from build123d import *

# Parameters (mm, degrees)
SALIENTE_EXTRUIR2_DEPTH = 3.2


with BuildPart() as part:
    # Croquis1 → Saliente-Extruir2 (new body)
    with BuildSketch(Plane(origin=(0, 0, 0), x_dir=(1, 0, 0), z_dir=(0, 1, 0))):
        with BuildLine():
            Line((-16.5, 3), (16.5, 3))
            ThreePointArc((16.5, 3), (20.541451884, 3.596020491), (24.238791177, 5.333333333))
            ThreePointArc((24.238791177, 5.333333333), (30.841182772, 8.435677694), (38.058061137, 9.5))
            Line((38.058061137, 9.5), (57.5, 9.5))
            Line((57.5, 9.5), (57.5, -9.5))
            Line((57.5, -9.5), (38.058061137, -9.5))
            ThreePointArc((38.058061137, -9.5), (30.841182772, -8.435677694), (24.238791177, -5.333333333))
            ThreePointArc((24.238791177, -5.333333333), (20.541451884, -3.596020491), (16.5, -3))
            Line((16.5, -3), (-16.5, -3))
            ThreePointArc((-16.5, -3), (-20.541451884, -3.596020491), (-24.238791177, -5.333333333))
            ThreePointArc((-24.238791177, -5.333333333), (-30.841182772, -8.435677694), (-38.058061137, -9.5))
            Line((-38.058061137, -9.5), (-57.5, -9.5))
            Line((-57.5, -9.5), (-57.5, 9.5))
            Line((-57.5, 9.5), (-38.058061137, 9.5))
            ThreePointArc((-38.058061137, 9.5), (-30.841182772, 8.435677694), (-24.238791177, 5.333333333))
            ThreePointArc((-24.238791177, 5.333333333), (-20.541451884, 3.596020491), (-16.5, 3))
        make_face()
    extrude(amount=SALIENTE_EXTRUIR2_DEPTH)


solid = part.part
Verification items for the finished model (mm, model axes). A direction names the side the tool comes from. Give positions to 0.01 mm unless a question says otherwise; leave off trailing zeros. Order: outer loops, then holes, each group sorted by start corner. A loop starts at its lowest first (then second) coordinate and runs counter-clockwise, first axis right, second up. Notation, with made-up numbers: M -7.75,46 L -0.75,46 A20 cw -0.75,68 Z; hole C -28,-15.75 d11. An arc over 180 degrees is marked long. Answer as a JSON object with one key per item and string values. Group by question number.
1) Depth check by flat-ended pin: pin 1 Ø3 at (x, z) = (15.5, -6) entering from -Y. Enter the tip coordinate at first touch or a pass-through.
2) Cross-section at D-D (x = 19.5). Enter the section's corners in (y, z).
3) Cross-section at B-B (y = 1.25). Enter the section's corners in (x, z), then the cut area to 3 significant figures.
4) Cross-section at C-C (z = 7.75). Enter the section's corners in (x, y).
5) Cross-section at A-A (z = -6.75). Enter the section's corners in (x, y).
6) Scan lines: line 1 along X through (y, z) = (0.95, 5.5); line 2 along Z through (x, y) = (3, 2.65); line 3 along X through (y, z) = (2.8, 5). Record each from-to range of solid material in increasing order. Write a range as [from, to].
7) Access from +Z, -Z, +X, -X, +Y, -Y to the whole of each face (thin tool, end or side, straight path). Record for faces 1 (the face through (-30.743, 1.578, 8.406)), 2 (the face through (48, 2, 9.5)), 3 (the face through (0, 2, -3)).
Result sheet:
{
 "1": {"pin 1": "passes through"},
 "2": {"outline": "M 0,-3.33 L 3.2,-3.33 L 3.2,3.33 L 0,3.33 Z"},
 "3": {"outline": "M -57.5,-9.5 L -38.06,-9.5 A25 ccw -24.24,-5.33 A14 cw -16.5,-3 L 16.5,-3 A14 cw 24.24,-5.33 A25 ccw 38.06,-9.5 L 57.5,-9.5 L 57.5,9.5 L 38.06,9.5 A25 ccw 24.24,5.33 A14 cw 16.5,3 L -16.5,3 A14 cw -24.24,5.33 A25 ccw -38.06,9.5 L -57.5,9.5 Z", "area": "1,500 mm2"},
 "4": {"outline": "M -57.5,0 L -28.87,0 L -28.87,3.2 L -57.5,3.2 Z; M 28.87,0 L 57.5,0 L 57.5,3.2 L 28.87,3.2 Z"},
 "5": {"outline": "M -57.5,0 L -26.66,0 L -26.66,3.2 L -57.5,3.2 Z; M 26.66,0 L 57.5,0 L 57.5,3.2 L 26.66,3.2 Z"},
 "6": {"line 1": "x = [-57.5, -24.49], [24.49, 57.5]", "line 2": "z = [-3, 3]", "line 3": "x = [-57.5, -23.71], [23.71, 57.5]"},
 "7": {"face 1": "+Z, +Y, -Y", "face 2": "+Z, +X, -X, +Y, -Y", "face 3": "-Z, +Y, -Y"}
}
